For this review, take the finished solid that the model builds, in its own axes (mm). Face numbers are marked on the shaded views. A direction names the side the tool comes from. Coordinates: 2 decimals unless noted, no trailing zeros. Order: outer loops, then holes, each group sorted by start corner. A loop starts at its lowest first (then second) coordinate and runs counter-clockwise, first axis right, second up. Notation, with made-up numbers: (72.5, 28.5) -> (106.5, 28.5) arc R21 cw to (106.5, 66.5) -> close; hole circle Ø3 at (6, -29.5). An arc over 180 degrees is marked (long way). Return JSON: item names as keys, results as strings. Group by question number.
Item 1: Insertion check: pin 1 (4 mm diameter, centred on x = -4.5, z = 7.5, fed in from +Y); pin 2 (3 mm diameter, centred on y = 2, z = 19.5, fed in from -X); pin 3 (1 mm diameter, centred on x = -0.5, y = 28.5, fed in from -Z); pin 4 (18 mm diameter, centred on y = 29.5, z = 24.5, fed in from -X). Each pin has a flat end and moves straight along its axis. Give the tip position at first contact, or say it passes through.
Item 2: For line 1 along X through (y, z) = (1.2, 35); line 2 along Y through (x, z) = (2.25, 30); line 3 along X through (y, z) = (37, -35), list the stretches that pass through material, from the lowest coordinate up.
Item 3: Take a section at D-D (y = 20.5). Write out the cut boundary in (x, z), then the cut area to 3 significant figures.
Item 4: Machinability: for the marked faces 1, 2 and 3, which of the approach directions +Z, -Z, +X, -X, +Y, -Y give a long, thin tool a straight path to every point of the face, cutting with its end or side? Answer none if there is none.
Item 5: Take a section at B-B (z = 35). Write out the cut boundary in (x, y).
Item 6: Take a section at C-C (y = 15). Write out the cut boundary in (x, z), then the cut area to 3 significant figures.
Item 7: Take a section at A-A (x = 0). Write out the cut boundary in (y, z), then the cut area to 3 significant figures.
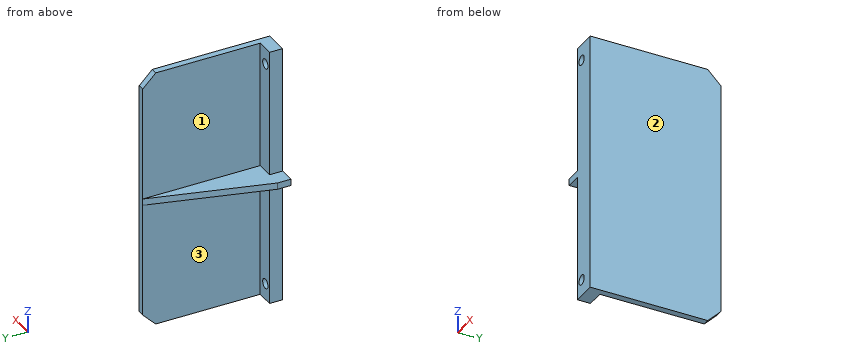
```python
from build123d import *

# Parameters (mm, degrees)
SKETCH_1_W      = 4.8
SKETCH_1_H      = 10
SKETCH_1_R      = 1.5
SKETCH_1_H_2    = 60
SKETCH_1_W_2    = 0.5
SKETCH_1_H_3    = 80
SKETCH_1_W_3    = 2
EXTRUDE_1_DEPTH = 4
SKETCH_1_4_W    = 2
SKETCH_1_4_H    = 80
EXTRUDE_3_DEPTH = 40
EXTRUDE_START   = -1
EXTRUDE_4_DEPTH = 2
CHAMFER_1_SIZE  = 4


# Read off the part's stored shape, not the designer's step: the extrude step
with BuildPart() as part:
    # Sketch 1 → Extrude 1 (new body)
    # profile 1 of 5: a face of its own
    with BuildSketch(Plane(origin=(0, 0, 0), x_dir=(1, 0, 0), z_dir=(0, 1, 0))):
        with Locations((0, -35)):
            Rectangle(SKETCH_1_W, SKETCH_1_H)
        with Locations(Location((0, -35, 0), (0, 0, 270))):
            Circle(SKETCH_1_R, mode=Mode.SUBTRACT)
    # profile 2 of 5: a face of its own
    with BuildSketch(Plane(origin=(0, 0, 0), x_dir=(1, 0, 0), z_dir=(0, 1, 0))):
        Rectangle(SKETCH_1_W, SKETCH_1_H_2)
    # profile 3 of 5: a face of its own
    with BuildSketch(Plane(origin=(0, 0, 0), x_dir=(1, 0, 0), z_dir=(0, 1, 0))):
        with Locations((0, 35)):
            Rectangle(SKETCH_1_W, SKETCH_1_H)
        with Locations(Location((0, 35, 0), (0, 0, 270))):
            Circle(SKETCH_1_R, mode=Mode.SUBTRACT)
    # profile 4 of 5: a face of its own
    with BuildSketch(Plane(origin=(0, 0, 0), x_dir=(1, 0, 0), z_dir=(0, 1, 0))):
        with Locations((2.65, 0)):
            Rectangle(SKETCH_1_W_2, SKETCH_1_H_3)
    # profile 5 of 5: a face of its own
    with BuildSketch(Plane(origin=(0, 0, 0), x_dir=(1, 0, 0), z_dir=(0, 1, 0))):
        with Locations((3.9, 0)):
            Rectangle(SKETCH_1_W_3, SKETCH_1_H_3)
    extrude(amount=EXTRUDE_1_DEPTH)

    # Sketch 1_4 → Extrude 3 (add)
    with BuildSketch(Plane(origin=(0, 0, 0), x_dir=(1, 0, 0), z_dir=(0, 1, 0))):
        with Locations((3.9, 0)):
            Rectangle(SKETCH_1_4_W, SKETCH_1_4_H)
    extrude(amount=EXTRUDE_3_DEPTH)

    # Extrude 4 outline → Extrude 4 (add)
    with BuildSketch(Plane.XY.offset(EXTRUDE_START)):
        Polygon((-7.1, 0), (-2.4, 0), (-2.4, 4), (2.9, 4), (2.9, 40), (-7.1, 4), align=None)
    extrude(amount=EXTRUDE_4_DEPTH)

    # Chamfer 1
    chamfer_1_edges = [part.edges().sort_by_distance(p)[0] for p in [
        (3.9, 40, -40),
        (3.9, 40, 40),
    ]]
    chamfer(chamfer_1_edges, length=CHAMFER_1_SIZE)


solid = part.part
```
Findings below:
{
 "1": {"pin 1": "passes through", "pin 2": "stops at x = -2.4", "pin 3": "stops at z = -1", "pin 4": "stops at x = 2.9"},
 "2": {"line 1": "x = -2.4 to -1.5, 1.5 to 4.9", "line 2": "y = 0 to 4", "line 3": "x = 2.9 to 4.9"},
 "3": {"outline": "(-2.52, -1) -> (2.9, -1) -> (2.9, -40) -> (4.9, -40) -> (4.9, 40) -> (2.9, 40) -> (2.9, 1) -> (-2.52, 1) -> close", "area": "171 mm2"},
 "4": {"face 1": "+Z, -X, +Y", "face 2": "+Z, -Z, +X, +Y, -Y", "face 3": "-Z, -X, +Y"},
 "5": {"outline": "(-2.4, 0) -> (-1.5, 0) -> (-1.5, 4) -> (-2.4, 4) -> close; (1.5, 0) -> (4.9, 0) -> (4.9, 40) -> (2.9, 40) -> (2.9, 4) -> (1.5, 4) -> close"},
 "6": {"outline": "(-4.04, -1) -> (2.9, -1) -> (2.9, -40) -> (4.9, -40) -> (4.9, 40) -> (2.9, 40) -> (2.9, 1) -> (-4.04, 1) -> close", "area": "174 mm2"},
 "7": {"outline": "(0, -40) -> (4, -40) -> (4, -36.5) -> (0, -36.5) -> close; (0, -33.5) -> (4, -33.5) -> (4, -1) -> (29.56, -1) -> (29.56, 1) -> (4, 1) -> (4, 33.5) -> (0, 33.5) -> close; (0, 36.5) -> (4, 36.5) -> (4, 40) -> (0, 40) -> close", "area": "347 mm2"}
}
